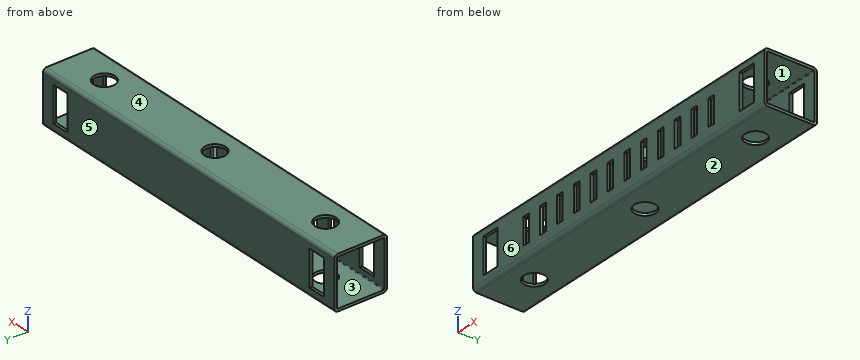
```python
from build123d import *

# Parameters (mm, degrees)
EXTRUDE_1_DEPTH            = 208
SKETCH_3_W                 = 8
SKETCH_3_H                 = 30
CUT_EXTRUDE_1_DEPTH        = 3
PATTERN_LINEAR_1_COUNT     = 6
PATTERN_LINEAR_1_PITCH     = 24
PATTERN_LINEAR_1_COL_COUNT = 7
PATTERN_LINEAR_1_COL_PITCH = 24
CUT_EXTRUDE_2_REACH        = 220.55
SKETCH_5_W                 = 20.5
SKETCH_5_H                 = 40.5
CUT_EXTRUDE_5_REACH        = 220.55
SKETCH_10_R                = 12.1


with BuildPart() as part:
    # Эскиз1 → Бобышка-Вытянуть1 (new, symmetric)
    with BuildSketch(Plane(origin=(0, 0, 0), x_dir=(0, 0, -1), z_dir=(1, 0, 0))):
        with BuildLine():
            Line((-26, -30), (26, -30))
            ThreePointArc((26, -30), (28.828427125, -28.828427125), (30, -26))
            Line((30, -26), (30, 26))
            ThreePointArc((30, 26), (28.828427125, 28.828427125), (26, 30))
            Line((26, 30), (-26, 30))
            ThreePointArc((-26, 30), (-28.828427125, 28.828427125), (-30, 26))
            Line((-30, 26), (-30, -26))
            ThreePointArc((-30, -26), (-28.828427125, -28.828427125), (-26, -30))
        make_face()
        with BuildLine():
            Line((-26, 27), (26, 27))
            ThreePointArc((26, 27), (26.707106781, 26.707106781), (27, 26))
            Line((27, 26), (27, -26))
            ThreePointArc((27, -26), (26.707106781, -26.707106781), (26, -27))
            Line((26, -27), (-26, -27))
            ThreePointArc((-26, -27), (-26.707106781, -26.707106781), (-27, -26))
            Line((-27, -26), (-27, 26))
            ThreePointArc((-27, 26), (-26.707106781, 26.707106781), (-26, 27))
        make_face(mode=Mode.SUBTRACT)
    extrude(amount=EXTRUDE_1_DEPTH, both=True)

    # Эскиз3 → Вырез-Вытянуть1 (cut)
    with BuildSketch(Plane.XZ.offset(30)):
        with Locations((-12, -1)):
            Rectangle(SKETCH_3_W, SKETCH_3_H)
    cut_extrude_1 = extrude(amount=-CUT_EXTRUDE_1_DEPTH, mode=Mode.SUBTRACT)

    # Линейный массив1: Вырез-Вытянуть1 ×6
    with Locations(*[(-i * PATTERN_LINEAR_1_PITCH, 0, 0) for i in range(1, PATTERN_LINEAR_1_COUNT)]):
        add(cut_extrude_1, mode=Mode.SUBTRACT)

    # Линейный массив1 col: Вырез-Вытянуть1 ×7
    with Locations(*[(i * PATTERN_LINEAR_1_COL_PITCH, 0, 0) for i in range(1, PATTERN_LINEAR_1_COL_COUNT)]):
        add(cut_extrude_1, mode=Mode.SUBTRACT)

    # Вырез-Вытянуть2: up to this face of the body (flat: up to its plane)
    cut_extrude_2_end = Plane(part.part.faces().sort_by_distance((0, 30, 0))[0])
    # Эскиз5 → Вырез-Вытянуть2 (cut, up to the picked face)
    with BuildSketch(Plane.XZ.offset(30), mode=Mode.PRIVATE) as cut_extrude_2_sk1:
        with Locations((-183, 0)):
            Rectangle(SKETCH_5_W, SKETCH_5_H)
    cut_extrude_2_tool1 = split(extrude(cut_extrude_2_sk1.sketch, amount=-CUT_EXTRUDE_2_REACH, mode=Mode.PRIVATE), bisect_by=cut_extrude_2_end, keep=Keep.BOTH, mode=Mode.PRIVATE)
    # Эскиз5 → Вырез-Вытянуть2 (cut, up to the picked face)
    with BuildSketch(Plane.XZ.offset(30), mode=Mode.PRIVATE) as cut_extrude_2_sk2:
        with Locations((183, 0)):
            Rectangle(SKETCH_5_W, SKETCH_5_H)
    cut_extrude_2_tool2 = split(extrude(cut_extrude_2_sk2.sketch, amount=-CUT_EXTRUDE_2_REACH, mode=Mode.PRIVATE), bisect_by=cut_extrude_2_end, keep=Keep.BOTH, mode=Mode.PRIVATE)
    add(cut_extrude_2_tool1.solids().sort_by(Axis((-183, -30, 0), (0, 1, 0)))[0], mode=Mode.SUBTRACT)
    add(cut_extrude_2_tool2.solids().sort_by(Axis((183, -30, 0), (0, 1, 0)))[0], mode=Mode.SUBTRACT)

    # Вырез-Вытянуть5: up to this face of the body (flat: up to its plane)
    cut_extrude_5_end = Plane(part.part.faces().sort_by_distance((0, 0, 30))[0])
    # Эскиз10 → Вырез-Вытянуть5 (cut, up to the picked face)
    with BuildSketch(Plane(origin=(0, 0, -30), x_dir=(-1, 0, 0), z_dir=(0, 0, -1)), mode=Mode.PRIVATE) as cut_extrude_5_sk1:
        with Locations(Location((-158, 0, 0), (0, 0, 90))):
            Circle(SKETCH_10_R)
    cut_extrude_5_tool1 = split(extrude(cut_extrude_5_sk1.sketch, amount=-CUT_EXTRUDE_5_REACH, mode=Mode.PRIVATE), bisect_by=cut_extrude_5_end, keep=Keep.BOTH, mode=Mode.PRIVATE)
    # Эскиз10 → Вырез-Вытянуть5 (cut, up to the picked face)
    with BuildSketch(Plane(origin=(0, 0, -30), x_dir=(-1, 0, 0), z_dir=(0, 0, -1)), mode=Mode.PRIVATE) as cut_extrude_5_sk2:
        with Locations(Location((158, 0, 0), (0, 0, 270))):
            Circle(SKETCH_10_R)
    cut_extrude_5_tool2 = split(extrude(cut_extrude_5_sk2.sketch, amount=-CUT_EXTRUDE_5_REACH, mode=Mode.PRIVATE), bisect_by=cut_extrude_5_end, keep=Keep.BOTH, mode=Mode.PRIVATE)
    # Эскиз10 → Вырез-Вытянуть5 (cut, up to the picked face)
    with BuildSketch(Plane(origin=(0, 0, -30), x_dir=(-1, 0, 0), z_dir=(0, 0, -1)), mode=Mode.PRIVATE) as cut_extrude_5_sk3:
        with Locations(Location((0, 0, 0), (0, 0, 90))):
            Circle(SKETCH_10_R)
    cut_extrude_5_tool3 = split(extrude(cut_extrude_5_sk3.sketch, amount=-CUT_EXTRUDE_5_REACH, mode=Mode.PRIVATE), bisect_by=cut_extrude_5_end, keep=Keep.BOTH, mode=Mode.PRIVATE)
    add(cut_extrude_5_tool1.solids().sort_by(Axis((158, 0, -30), (0, 0, 1)))[0], mode=Mode.SUBTRACT)
    add(cut_extrude_5_tool2.solids().sort_by(Axis((-158, 0, -30), (0, 0, 1)))[0], mode=Mode.SUBTRACT)
    add(cut_extrude_5_tool3.solids().sort_by(Axis((0, 0, -30), (0, 0, 1)))[0], mode=Mode.SUBTRACT)


solid = part.part
```
Part model, mm, in its own coordinate system. Face numbers are marked on the shaded views. A direction names the side the tool comes from. Round coordinates to 2 decimals unless told otherwise and drop trailing zeros. Order: outer loops, then holes, each group sorted by start corner. A loop starts at its lowest first (then second) coordinate and runs counter-clockwise, first axis right, second up. Notation, with made-up numbers: M 31,-6 L 82,-6 A28 cw 82,28 Z; hole C 32,-25.75 d8. An arc over 180 degrees is marked long. Answer in a Markdown table with one row per item. Add a question column.
Q1. Wall check: L1, parallel to X at y = 0, z = -29.1; L2, parallel to Z at x = 116, y = -22. Give the ranges that are in metal, low to high. Write a range as from..to.
Q2. 3-axis set-ups, long thin cutter, end or side, ignore diameter. For the marked faces 1 and 2: which of +Z, -Z, +X, -X, +Y, -Y reach the whole face in a straight line?
Q3. Mould opens along Y. For the marked faces 3, 4, 5 and 6 say: +Y half, -Y half, draft (parallel to the pull), parting line (faces both ways), or undercut.
Q4. Pin check, flat tips, straight feed: pin 1 (2.5 mm diameter, centred on x = -109, y = -29, fed in from +Z); pin 2 (3.5 mm diameter, centred on x = -37.5, y = -29, fed in from -Z); pin 3 (0.9 mm diameter, centred on x = 106.5, y = -28.5, fed in from +Z). Stop position of each tip, or through.
Q5. Cut at A-A on y = -17. Give the cut face in (x, z), and give its area (3 significant figures).
Q6. Cut at C-C on y = 0. Give the number of separate pieces and of enclosed holes in the cut face, and give its area (3 significant figures).
Q7. Cut at B-B on x = -158. Give the cut face in (y, z).
Q8. Cut at D-D on x = 115.5. Give the cut face in (y, z).
Established:
| question | item | result |
|---|---|---|
| 1 | L1 | x = -208..-170.1, -145.9..-12.1, 12.1..145.9, 170.1..208 |
| 1 | L2 | z = -30..-27, 27..30 |
| 2 | face 1 | +X, -X |
| 2 | face 2 | -Z, +X, -X, +Y, -Y |
| 3 | face 3 | undercut |
| 3 | face 4 | draft |
| 3 | face 5 | +Y half |
| 3 | face 6 | -Y half |
| 4 | pin 1 | stops at z = 29.6 |
| 4 | pin 2 | stops at z = -29.8 |
| 4 | pin 3 | stops at z = 29.43 |
| 5 | outline | M -208,-30 L 208,-30 L 208,-27 L -208,-27 Z; M -208,27 L 208,27 L 208,30 L -208,30 Z |
| 5 | area | 2,500 mm2 |
| 6 | separate pieces | 8 |
| 6 | enclosed holes | 0 |
| 6 | area | 2,060 mm2 |
| 7 | outline | M -30,-26 A4 ccw -26,-30 L -12.1,-30 L -12.1,-27 L -26,-27 A1 cw -27,-26 L -27,26 A1 cw -26,27 L -12.1,27 L -12.1,30 L -26,30 A4 ccw -30,26 Z; M 12.1,-30 L 26,-30 A4 ccw 30,-26 L 30,26 A4 ccw 26,30 L 12.1,30 L 12.1,27 L 26,27 A1 cw 27,26 L 27,-26 A1 cw 26,-27 L 12.1,-27 Z |
| 8 | outline | M -30,-26 A4 ccw -26,-30 L 26,-30 A4 ccw 30,-26 L 30,26 A4 ccw 26,30 L -26,30 A4 ccw -30,26 Z; hole M -27,-26 A1 ccw -26,-27 L 26,-27 A1 ccw 27,-26 L 27,26 A1 ccw 26,27 L -26,27 A1 ccw -27,26 Z |
